Design review of the part shown in the three views and the two pictorial views. Dimensions are in mm from the part's minimum x, y and z. A direction names the side the tool comes from. Coordinates: 2 decimals unless noted, no trailing zeros. Write each loop counter-clockwise with the first axis right and the second up, starting at its lowest first coordinate (ties: lowest second). Pieces come first, ordered by that corner, then holes. Notation, with made-up numbers: M 41,-37.75 L 81,-37.75 A30 cw 81,-0.75 Z; hole C 8.5,-2 d8. An arc over 180 degrees is marked long. Answer as a JSON object with one key per item and string values.
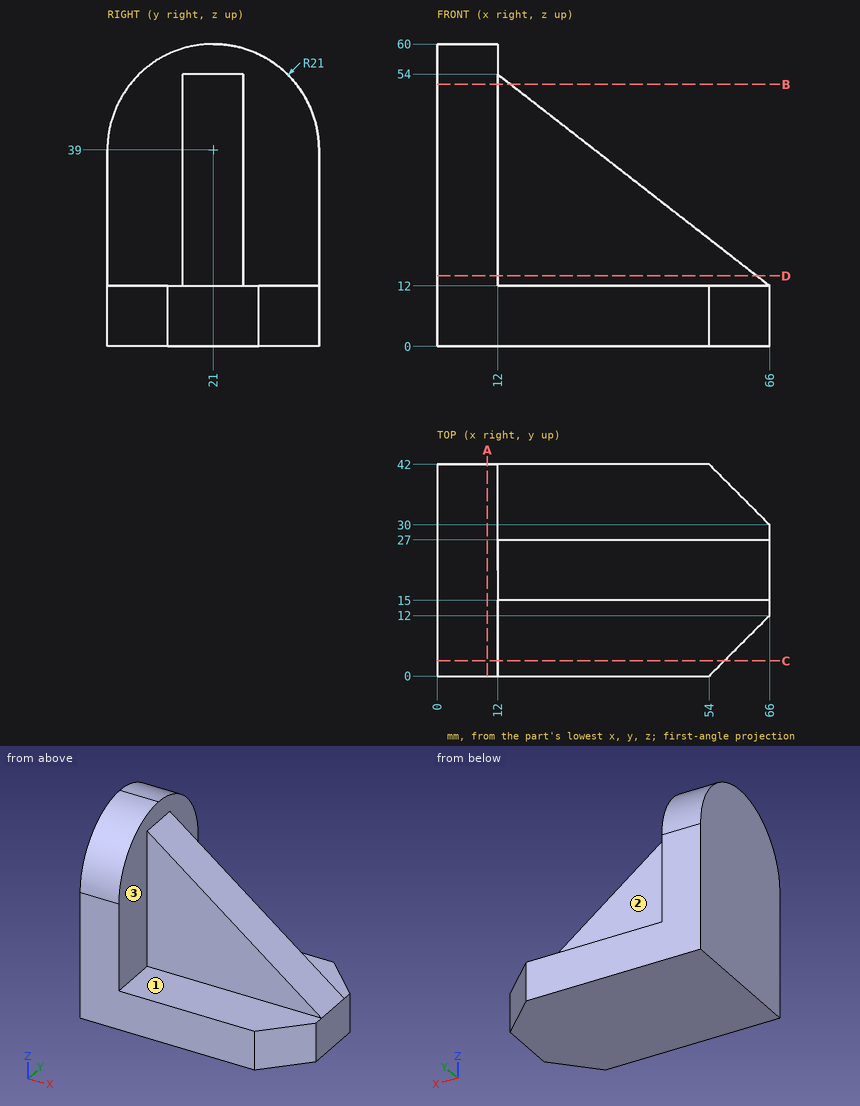
(1) For pin 1 Ø4 at (x, z) = (33.5, 27.5) entering from +Y; pin 2 Ø3 at (y, z) = (8, 34.5) entering from +X; pin 3 Ø16.5 at (x, y) = (46, 36.5) entering from +Z, all flat-tipped, find the tip position at first contact; note any pin that passes through.
Results list:
{"pin 1": "y = 27", "pin 2": "x = 12", "pin 3": "z = 12"}
(2) For the marked faces 1, 2 and 3, list the 3-axis set-ups (+Z, -Z, +X, -X, +Y, -Y) from which the entire face can be reached by the end or side of a thin tool; tool diameter is ignored.
Results list:
{"face 1": "+Z, +X, -Y", "face 2": "+Z, +X, +Y", "face 3": "+Z, +X"}
(3) Add section B-B on z = 52. Give the boundary of the cut face in (x, y), and give its area (3 significant figures).
Results list:
{"outline": "M 0,4.51 L 12,4.51 L 12,15 L 14.57,15 L 14.57,27 L 12,27 L 12,37.49 L 0,37.49 Z", "area": "427 mm²"}
(4) Wall thickness on line 1 along Z through (x, y) = (55, 5); line 2 along Y through (x, z) = (37, 26): over which ranges is each line inside the solid? List them lowest first. Write a range as from..to.
Results list:
{"line 1": "0..12", "line 2": "15..27"}
(5) Add section C-C on y = 3. Give the boundary of the cut face in (x, z).
Results list:
{"outline": "M 0,0 L 57,0 L 57,12 L 12,12 L 12,49.82 L 0,49.82 Z"}
(6) Add section A-A on x = 10. Give the boundary of the cut face in (y, z), and give its area (3 significant figures).
Results list:
{"outline": "M 0,0 L 42,0 L 42,39 A21 ccw 0,39 Z", "area": "2,330 mm²"}
(7) Add section D-D on z = 14. Give the boundary of the cut face in (x, y), and give its area (3 significant figures).
Results list:
{"outline": "M 0,0 L 12,0 L 12,15 L 63.43,15 L 63.43,27 L 12,27 L 12,42 L 0,42 Z", "area": "1,120 mm²"}
